The model under review builds one solid part; all positions refer to its coordinate system, in mm. A direction names the side the tool comes from. Coordinates: 2 decimals unless noted, no trailing zeros. Loops run counter-clockwise (first coordinate to the right, second up) from the corner with the lowest first, then second, coordinate; pieces in that order, holes last. Notation, with made-up numbers: M 40.25,88 L 84.25,88 A29 ccw 84.25,123 Z; hole C -36,37.5 d10. An arc over 180 degrees is marked long. One line per item, written item: value.
```python
from build123d import *

# Parameters (mm, degrees)
SKETCH4_R           = 8.5
SKETCH4_R_2         = 1.5
BOSS_EXTRUDE1_DEPTH = 3


with BuildPart() as part:
    # Sketch4 → Boss-Extrude1 (new body)
    with BuildSketch(Plane(origin=(0, 0, 0), x_dir=(1, 0, 0), z_dir=(0, 1, 0))):
        Polygon((-26, -90), (-9.5, -90), (-9.5, -87), (15.5, -87), (15.5, -90), (32, -90), (32, -78), (29, -78), (29, -56), (32, -56), (32, -34), (29, -34), (29, -12), (32, -12), (32, 0), (15.5, 0), (15.5, -3), (-9.5, -3), (-9.5, 0), (-26, 0), (-26, -12), (-23, -12), (-23, -34), (-26, -34), (-26, -56), (-23, -56), (-23, -78), (-26, -78), align=None)
        with Locations((-4.2, -20.197580763)):
            Circle(SKETCH4_R, mode=Mode.SUBTRACT)
        with Locations((-12, -45)):
            Circle(SKETCH4_R_2, mode=Mode.SUBTRACT)
    extrude(amount=BOSS_EXTRUDE1_DEPTH)


solid = part.part
```
(1) To check wall thickness, follow L1, parallel to X at y = 0.65, z = 45; L2, parallel to Z at x = -11.5, y = 1.9; L3, parallel to X at y = 1.1, z = 70.5. State the ranges of each line that lie inside material, in increasing order. Write a range as [from, to].
Checks:
L1: [-26, -13.5], [-10.5, 32]
L2: [0, 15.84], [24.55, 43.59], [46.41, 90]
L3: [-23, 29]
(2) Add section B-B on z = 45. State the section outline as (x, y) points.
Checks:
outline: M -26,0 L -13.5,0 L -13.5,3 L -26,3 Z; M -10.5,0 L 32,0 L 32,3 L -10.5,3 Z
(3) Tool access review of faces 1 (the face through (32, 1, 84)), 2 (the face through (-24, 1, 78)), 3 (the face through (3, 1, 3)), 4 (the face through (3, 0, 44)), 5 (the face through (31, 1, 34)): name each direction out of +Z, -Z, +X, -X, +Y, -Y from which nothing blocks a thin tool from reaching the whole face with its end or side.
Checks:
face 1: +Z, -Z, +X, +Y, -Y
face 2: -X, +Y, -Y
face 3: -Z, +Y, -Y
face 4: +Z, -Z, +X, -X, -Y
face 5: +X, +Y, -Y
(4) Add section A-A on x = -4.2. State the section outline as (y, z) points, then the cut area to 3 significant figures.
Checks:
outline: M 0,3 L 3,3 L 3,11.7 L 0,11.7 Z; M 0,28.7 L 3,28.7 L 3,87 L 0,87 Z
area: 201 mm^2
(5) Add section D-D on z = 62. State the section outline as (x, y) points.
Checks:
outline: M -23,0 L 29,0 L 29,3 L -23,3 Z
(6) Add section C-C on y = 1.35. State how many separate pieces and enclosed holes the cut face has, then the cut area to 3 significant figures.
Checks:
separate pieces: 1
enclosed holes: 2
area: 4,570 mm^2
(7) Draft analysis for pull direction X (two halves, no side actions). For faces 6 (the face through (3, 3, 44)), 7 (the face through (-23, 1, 23)), 8 (the face through (-9.5, 1, 89)), state which applies: pulls with the +X half, pulls with the -X half, needs draft (parallel to the pull), parting line crosses it, or undercut.
Checks:
face 6: needs draft
face 7: pulls with the -X half
face 8: undercut
(8) Insertion check: pin 1 Ø0.9 at (x, y) = (1, 1) entering from -Z; pin 2 Ø0.9 at (y, z) = (1.5, 19.5) entering from +X; pin 3 Ø1.5 at (x, y) = (8.5, 2) entering from +Z. Each pin has a flat end and moves straight along its axis. Give the tip position at first contact, or say it passes through.
Checks:
pin 1: z = 3
pin 2: x = 29
pin 3: z = 87
